Model file for the job. Use its own axes, mm. A direction names the side the tool comes from. Coordinates: 2 decimals unless noted, no trailing zeros. Write each loop counter-clockwise with the first axis right and the second up, starting at its lowest first coordinate (ties: lowest second). Pieces come first, ordered by that corner, then holes. Notation, with made-up numbers: M 43.25,30 L 60.25,30 A31 cw 60.25,58 Z; hole C 54.25,-18 d2. An arc over 180 degrees is marked long. Put each result on its own line as item: value. Start each with the question number.
Q1. Cut at B-B (z = 0). Write the cut outline in (x, y), then the cut area to 3 significant figures.
Q2. Drill centre lines: line 1 along X through (y, z) = (10.3, 0); line 2 along X through (y, z) = (0.75, 0.5); line 3 along Y through (x, z) = (-9, 3.5). Where is each one in solid material? Low to high.
Q3. Pull direction X, two halves, no side cores. Call faces 1 (the cylindrical face through (5.52, 9.46, 13.3)), 2 (the cylindrical face through (9.7, 5.5, -12.6)), 3 (the flat face through (-4, -2, 14)): pulls with the +X half, pulls with the -X half, needs draft (parallel to the pull), parting line crosses it, or undercut.
Q4. Which spindle directions (+Z, -Z, +X, -X, +Y, -Y) get a long thin tool onto all of the face, cutting with end or side? Do faces 4 (the flat face through (0, 1.5, 0)), 5 (the flat face through (6, 13, 14)), 6 (the flat face through (0, 0, 0)). Say none if no direction does.
Q5. Cut at A-A (x = 0). Write the cut outline in (y, z).
Q6. Cut at D-D (y = 0.5). Write the cut outline in (x, z), then the cut area to 3 significant figures.
Q7. Drop flat-ended pins along their axis: pin 1 (2 mm diameter, centred on y = 8, z = -10, fed in from +X); pin 2 (4 mm diameter, centred on x = 6.5, y = 7, fed in from +Z); pin 3 (12.5 mm diameter, centred on x = 5.5, z = -2.5, fed in from -Y). Give the stop position or say it passes through.
Q8. Cut at C-C (y = 10). Write the cut outline in (x, z).
```python
from build123d import *

# Parameters (mm, degrees)
CHAMFER1_SIZE = 0.5
CHAMFER2_SIZE = 0.2


with BuildPart() as part:
    # Sketch1 → Revolve1 (revolve)
    with BuildSketch(Plane.XY, mode=Mode.PRIVATE) as revolve1_sk:
        with BuildLine():
            Line((0, 0), (-12.4, 0))
            ThreePointArc((-12.4, 0), (-13.814213562, -0.585786438), (-14.4, -2))
            Line((-14.4, -2), (-15.9, -2))
            Line((-15.9, -2), (-15.9, 13))
            Line((-15.9, 13), (-14.4, 13))
            Line((-14.4, 13), (-14.4, 6.5))
            ThreePointArc((-14.4, 6.5), (-12.935533906, 2.964466094), (-9.4, 1.5))
            Line((-9.4, 1.5), (0, 1.5))
            Line((0, 1.5), (0, 0))
        make_face()
    revolve(revolve1_sk.sketch.rotate(Axis((0, 1.5, 0), (0, -1, 0)), 270), axis=Axis((0, 1.5, 0), (0, -1, 0)))

    # Chamfer1
    chamfer1_edges = [part.edges().sort_by_distance(p)[0] for p in [
        (0, 13, -14.4),
    ]]
    chamfer(chamfer1_edges, length=CHAMFER1_SIZE)

    # Chamfer2
    chamfer2_edges = [part.edges().sort_by_distance(p)[0] for p in [
        (0, 13, -15.9),
    ]]
    chamfer(chamfer2_edges, length=CHAMFER2_SIZE)


solid = part.part
```
Computed values:
1. outline: M -15.9,-2 L -14.4,-2 A2 cw -12.4,0 L 12.4,0 A2 cw 14.4,-2 L 15.9,-2 L 15.9,12.8 L 15.7,13 L 14.9,13 L 14.4,12.5 L 14.4,6.5 A5 cw 9.4,1.5 L -9.4,1.5 A5 cw -14.4,6.5 L -14.4,12.5 L -14.9,13 L -15.7,13 L -15.9,12.8 Z
1. area: 100 mm2
2. line 1: -15.9 to -14.4, 14.4 to 15.9
2. line 2: -15.89 to 15.89
2. line 3: 0 to 1.51
3. face 1: undercut
3. face 2: parting line crosses it
3. face 3: needs draft
4. face 4: +Y
4. face 5: +Z, -Z, +X, -X, +Y
4. face 6: -Y
5. outline: M -2,-15.9 L 12.8,-15.9 L 13,-15.7 L 13,-14.9 L 12.5,-14.4 L 6.5,-14.4 A5 cw 1.5,-9.4 L 1.5,9.4 A5 cw 6.5,14.4 L 12.5,14.4 L 13,14.9 L 13,15.7 L 12.8,15.9 L -2,15.9 L -2,14.4 A2 cw 0,12.4 L 0,-12.4 A2 cw -2,-14.4 Z
6. outline: C 0,0 d31.8
6. area: 794 mm2
7. pin 1: x = 13.11
7. pin 2: z = 15.25
7. pin 3: y = 0
8. outline: C 0,0 d31.8; hole C 0,0 d28.8
